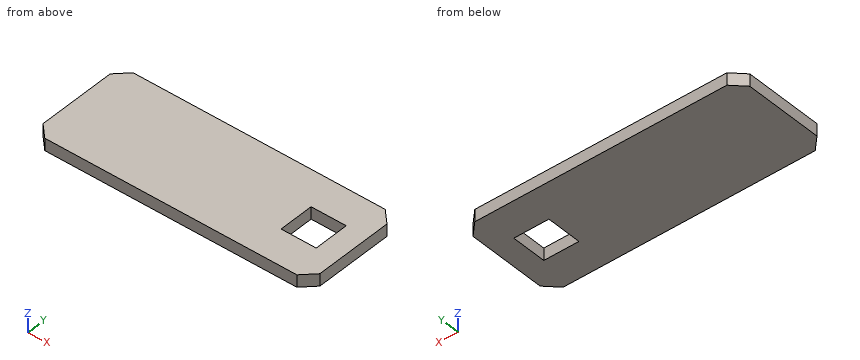
from build123d import *

# Parameters (mm, degrees)
SKETCH_1_W             = 84
SKETCH_1_H             = 55
SM_BASE_FLANGE_1_DEPTH = 2.95
SKETCH_5_W             = 8.5
SKETCH_5_H             = 8.5
CUT_EXTRUDE_1_DEPTH    = 10
CHAMFER_1_SIZE         = 3


# Sheet-metal steps are written as plain solids
with BuildPart() as part:
    # Sketch 1 → Базовая кромка1 (new body)
    with BuildSketch(Plane.XY):
        with Locations((-22.345696863, 3.516131621)):
            Rectangle(SKETCH_1_W, SKETCH_1_H)
    extrude(amount=-SM_BASE_FLANGE_1_DEPTH)

    # Эскиз5 → Вырез-Вытянуть1 (cut)
    with BuildSketch(Plane(origin=(0, 0, -2.95), x_dir=(-1, 0, 0), z_dir=(0, 0, -1))):
        Polygon((64.345696863, -23.983868379), (64.345696863, -8.483868379), (-2.654303137, -8.483868379), (-2.654303137, 16.516131621), (64.345696863, 16.516131621), (64.345696863, 31.016131621), (-19.654303137, 31.016131621), (-19.654303137, -23.983868379), align=None)
        with Locations((6.948166656, 3.987990807)):
            Rectangle(SKETCH_5_W, SKETCH_5_H)
    extrude(amount=-CUT_EXTRUDE_1_DEPTH, mode=Mode.SUBTRACT)

    # Фаска1
    chamfer_1_edges = [part.edges().sort_by_distance(p)[0] for p in [
        (2.654303137, 16.516131621, -1.475),
        (2.654303137, -8.483868379, -1.475),
        (-64.345696863, -8.483868379, -1.475),
        (-64.345696863, 16.516131621, -1.475),
    ]]
    chamfer(chamfer_1_edges, length=CHAMFER_1_SIZE)


solid = part.part
Input: part model. Units: mm. Frame: model coordinates. Give positions to 0.01 mm unless a question says otherwise; leave off trailing zeros. Loops run counter-clockwise (first coordinate to the right, second up) from the corner with the lowest first, then second, coordinate; pieces in that order, holes last. Notation, with made-up numbers: M -4,83 L 21,83 A8 ccw 21,93 Z; hole C 89.5,6.5 d6. An arc over 180 degrees is marked long. Use one line per item in the form item = value.
1. Line query: L1, parallel to X at y = 7, z = -1.75; L2, parallel to Y at x = -10, z = -0.1; L3, parallel to X at y = 15.25, z = -0.95. Output: solid intervals per line, ascending.
Numbers:
L1 = -64.35 to -11.2, -2.7 to 2.65
L2 = -8.48 to -0.26, 8.24 to 16.52
L3 = -62.61 to 0.92
2. Section query B-B, the plane z = -2.1. Return the cut outline in (x, y).
Numbers:
outline = M -64.35,-5.48 L -61.35,-8.48 L -0.35,-8.48 L 2.65,-5.48 L 2.65,13.52 L -0.35,16.52 L -61.35,16.52 L -64.35,13.52 Z; hole M -11.2,-0.26 L -2.7,-0.26 L -2.7,8.24 L -11.2,8.24 Z
3. Section query C-C, the plane y = -6.75. Return the cut outline in (x, z).
Numbers:
outline = M -63.08,-2.95 L 1.39,-2.95 L 1.39,0 L -63.08,0 Z
4. Section query A-A, the plane y = 1.25. Return the cut outline in (x, z).
Numbers:
outline = M -64.35,-2.95 L -11.2,-2.95 L -11.2,0 L -64.35,0 Z; M -2.7,-2.95 L 2.65,-2.95 L 2.65,0 L -2.7,0 Z
